Could you check a few things on this drawing? It's one solid part, dimensions in mm from its lowest x, y, z. A direction names the side the tool comes from. Give positions to 0.01 mm unless a question says otherwise; leave off trailing zeros. Order: outer loops, then holes, each group sorted by start corner. A loop starts at its lowest first (then second) coordinate and runs counter-clockwise, first axis right, second up.
Item 1: I want a section at C-C, the plane x = 157.5. Write out the boundary of the cut face in (y, z), then the cut area to 3 significant figures.
Item 2: I'm going to push flat-ended pins straight in: pin 1 Ø10 at (y, z) = (127, 32) entering from +X; pin 2 Ø8 at (y, z) = (204, 12.5) entering from -X; pin 3 Ø6 at (x, z) = (569.5, 69) entering from +Y. Where does each tip first touch, or does it pass through?
Item 3: If we mould it in two halves opening along X, with no side actions, what happens to the marked faces 1 and 2? For each: +X half, -X half, draft (parallel to the pull), parting line (faces both ways), or undercut.
Item 4: If I drill on line 1 along Y through (x, z) = (364, 40); line 2 along X through (y, z) = (364, 62); line 3 along Y through (x, z) = (291.5, 74.5) (1 decimal), over which ranges is the centre line in solid material (lowest first)?
Item 5: I want a section at B-B, the plane y = 637. Write out the boundary of the cut face in (x, z), then the cut area to 3 significant figures.
Item 6: Which directions (+Z, -Z, +X, -X, +Y, -Y) give clear straight access to the entire face, cutting with the end or side of a thin tool? Please do the marked faces 3 and 4.
Item 7: I want a section at A-A, the plane z = 51. Write out the boundary of the cut face in (x, y).
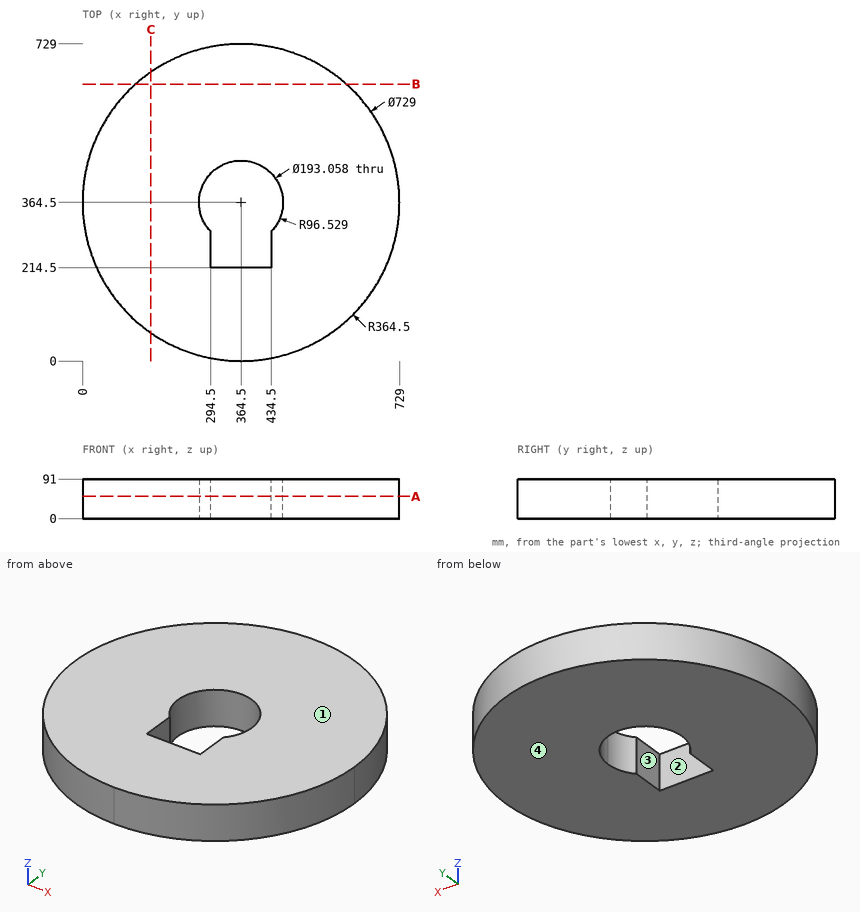
Results list:
1. outline: (64.48, 0) - (664.52, 0) - (664.52, 91) - (64.48, 91) - close
1. area: 54,600 mm2
2. pin 1: stops at x = 645.22
2. pin 2: stops at x = 35.31
2. pin 3: stops at y = 667.91
3. face 1: draft
3. face 2: undercut
4. line 1: y = 0 to 214.5, 461.03 to 729
4. line 2: x = 0 to 267.97, 461.03 to 729
4. line 3: y = 7.4 to 301.3, 427.7 to 721.6
5. outline: (122.42, 0) - (606.58, 0) - (606.58, 91) - (122.42, 91) - close
5. area: 44,100 mm2
6. face 3: +Z, -Z
6. face 4: -Z, +X, -X, +Y, -Y
7. outline: circle Ø729 at (364.5, 364.5); hole (294.5, 214.5) - (434.5, 214.5) - (434.5, 298.03) arc R96.53 ccw (long way) to (294.5, 298.03) - close
